Input: part model. Units: mm. Frame: model coordinates. A direction names the side the tool comes from. Coordinates: 2 decimals unless noted, no trailing zeros. Order: outer loops, then holes, each group sorted by start corner. A loop starts at its lowest first (then second) coordinate and runs counter-clockwise, first axis right, second up. Notation, with made-up numbers: (-4.75, -30.5) -> (10.25, -30.5) arc R14 ccw to (10.25, -9.5) -> close; hole circle Ø9 at (42.25, -4.75). An arc over 180 degrees is marked (long way). Write each question's results on one line, items separated by ' | '.
```python
from build123d import *

# Parameters (mm, degrees)
F0_R     = 8.5
F1_DEPTH = 8
F2_R     = 3.8
F3_DEPTH = 2
F4_R     = 2.5
F5_DEPTH = 10.001
F6_R     = 3
F8_R     = 3.8
F8_R_2   = 2.5
F9_DEPTH = 1


with BuildPart() as f1:
    # F0 (on Top) → F1 (new body)
    with BuildSketch(Plane.XY):
        Circle(F0_R)
    extrude(amount=F1_DEPTH)

    # F2 (on face) → F3 (join)
    with BuildSketch(Plane.XY.offset(8)):
        Circle(F2_R)
    extrude(amount=F3_DEPTH)

    # F4 (on face) → F5 (cut, through all)
    with BuildSketch(Plane.XY.offset(10)):
        Circle(F4_R)
    extrude(amount=-F5_DEPTH, mode=Mode.SUBTRACT)

    # F6 (on Right) → F7 (revolve, cut)
    with BuildSketch(Plane.YZ):
        with Locations((-10.25, 4)):
            Circle(F6_R)
    revolve(axis=Axis((0, 0, 7.899270393), (0, 0, 1)), mode=Mode.SUBTRACT)

    # F8 (on face) → F9 (cut)
    with BuildSketch(Plane(origin=(0, 0, 0), x_dir=(1, 0, 0), z_dir=(0, 0, -1))):
        Circle(F8_R)
        Circle(F8_R_2, mode=Mode.SUBTRACT)
    extrude(amount=-F9_DEPTH, mode=Mode.SUBTRACT)


solid = f1.part
```
(1) Line query: line 1 along Y through (x, z) = (0, 0.6); line 2 along X through (y, z) = (0, 6.5); line 3 along Y through (x, z) = (0, 3). Output: solid intervals per line, ascending. Write a range as from..to.
Return value:
line 1: -8.5..-3.8, 3.8..8.5 | line 2: -8.5..-2.5, 2.5..8.5 | line 3: -7.42..-2.5, 2.5..7.42
(2) Cut plane D-D, the plane z = 7. Return loops of the section in (x, y), plus the area to 3 significant figures.
Return value:
outline: circle Ø17 at (0, 0); hole circle Ø5 at (0, 0) | area: 207 mm2
(3) Mould query, pull axis Y, two halves, no side actions, for faces 4 (the face through (4.57, 7.167, 0.771)), 5 (the face through (-0.54, -2.44, 5.56)), 6 (the face through (-0.9, -2.5, 10)). Classes: +Y half, -Y half, draft (parallel to the pull), parting line (faces both ways), or undercut.
Return value:
face 4: parting line | face 5: undercut | face 6: draft
(4) Pin query (flat end, axial travel): P1, Ø4, axis at x = -3.5, y = -6, coming from the +Z side; P2, Ø4, axis at x = -4, z = 8.5, coming from the -Y side; P3, Ø3, axis at x = -4.5, z = 3, coming from the -Y side (3 decimals). Return the tip coordinate at first contact, or that it passes through.
Return value:
P1: z = 8 | P2: y = -8.25 | P3: y = -7.465
(5) Cut plane C-C, the plane z = 9.25. Return loops of the section in (x, y), plus the area to 3 significant figures.
Return value:
outline: circle Ø7.6 at (0, 0); hole circle Ø5 at (0, 0) | area: 25.7 mm2
(6) Cut plane A-A, the plane x = 0. Return loops of the section in (y, z).
Return value:
outline: (-8.5, 0) -> (-3.8, 0) -> (-3.8, 1) -> (-2.5, 1) -> (-2.5, 10) -> (-3.8, 10) -> (-3.8, 8) -> (-8.5, 8) -> (-8.5, 6.44) arc R3 cw to (-8.5, 1.56) -> close; (2.5, 1) -> (3.8, 1) -> (3.8, 0) -> (8.5, 0) -> (8.5, 1.56) arc R3 cw to (8.5, 6.44) -> (8.5, 8) -> (3.8, 8) -> (3.8, 10) -> (2.5, 10) -> close
(7) Reachability of faces 1 (the face through (-3.796, 0.167, 8.986)), 2 (the face through (4, -2, 0)), 3 (the face through (-3.796, -0.167, 0.493)) from +Z, -Z, +X, -X, +Y, -Y: full face, straight path, thin tool, end or side. Return the list, or none.
Return value:
face 1: +Z | face 2: -Z, +X, -X, +Y, -Y | face 3: -Z
